Could you check a few things on this drawing? It's one solid part, dimensions in mm from its lowest x, y, z. Round coordinates to 2 decimals unless told otherwise and drop trailing zeros. Write each loop counter-clockwise with the first axis right and the second up, starting at its lowest first coordinate (ties: lowest second). Pieces come first, ordered by that corner, then holes. Notation, with made-up numbers: (66, -23.5) -> (123, -23.5) arc R8 ccw to (123, -13.5) -> close; hole circle Ø4 at (-20, 49). An arc over 180 degrees is marked (long way). Answer as CSV lines item,"result".
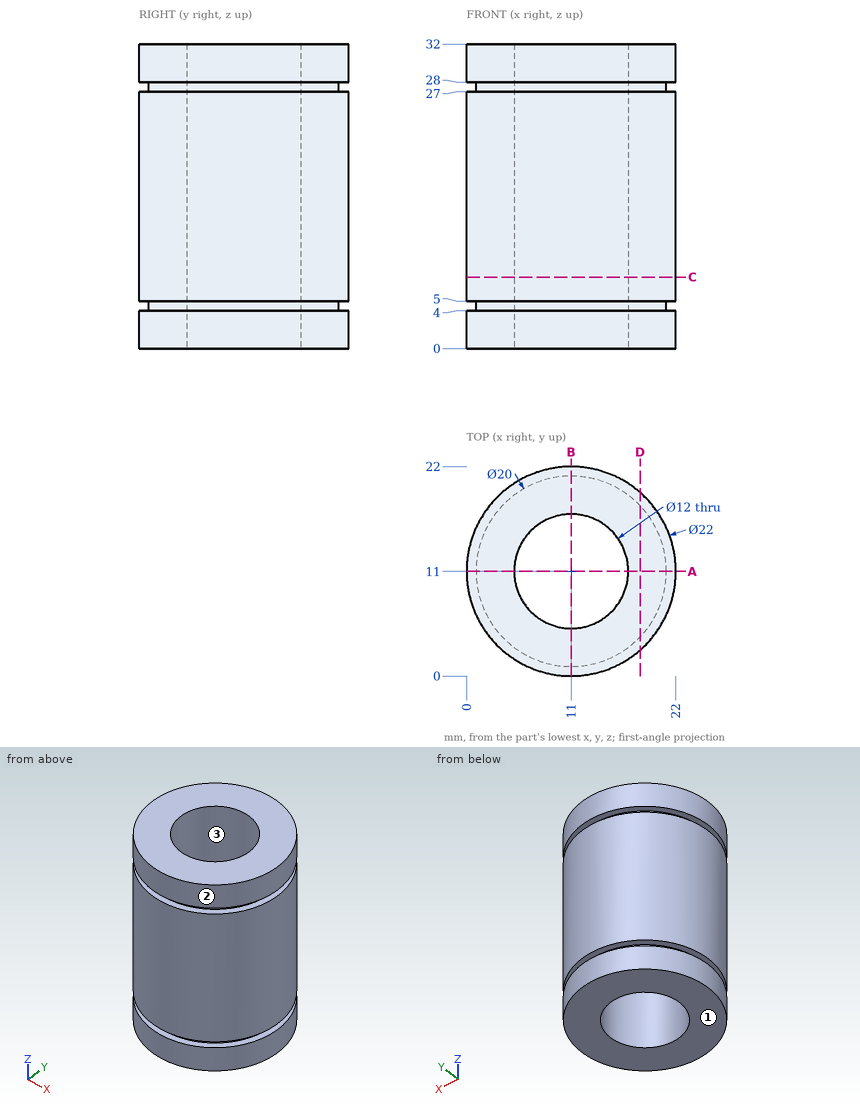
1. For pin 1 Ø12 at (y, z) = (3.5, 9) entering from -X; pin 2 Ø4 at (y, z) = (7, 10.5) entering from +X; pin 3 Ø6.5 at (x, y) = (10, 12) entering from -Z; pin 4 Ø1.5 at (x, z) = (3.5, 25) entering from +Y, each with a flat end and sliding along its axis, tell me the tip position at first contact or that it passes through.
Numbers:
pin 1,"stops at x = 0.1"
pin 2,"stops at x = 21.82"
pin 3,"passes through"
pin 4,"stops at y = 19.69"
2. If I drill on line 1 (Y direction, x = 11, z = 18.5); line 2 (Y direction, x = 15.75, z = 8); line 3 (X direction, y = 6.5, z = 19.5), over which ranges is the centre line in solid material (lowest first)?
Numbers:
line 1,"y = 0 to 5, 17 to 22"
line 2,"y = 1.08 to 7.33, 14.67 to 20.92"
line 3,"x = 0.96 to 7.03, 14.97 to 21.04"
3. If we mould it in two halves opening along X, with no side actions, what happens to the marked faces 1, 2 and 3? For each: released by +X, released by -X, zero draft, split by the parting line, or undercut.
Numbers:
face 1,"zero draft"
face 2,"split by the parting line"
face 3,"undercut"
4. Suppose I cut it at D-D on x = 18.25. Please give me the cut outline in (y, z), and give its area (3 significant figures).
Numbers:
outline,"(2.73, 0) -> (19.27, 0) -> (19.27, 4) -> (17.89, 4) -> (17.89, 5) -> (19.27, 5) -> (19.27, 27) -> (17.89, 27) -> (17.89, 28) -> (19.27, 28) -> (19.27, 32) -> (2.73, 32) -> (2.73, 28) -> (4.11, 28) -> (4.11, 27) -> (2.73, 27) -> (2.73, 5) -> (4.11, 5) -> (4.11, 4) -> (2.73, 4) -> close"
area,"524 mm^2"
5. Suppose I cut it at A-A on y = 11. Please give me the cut outline in (x, z), and give its area (3 significant figures).
Numbers:
outline,"(0, 0) -> (5, 0) -> (5, 32) -> (0, 32) -> (0, 28) -> (1, 28) -> (1, 27) -> (0, 27) -> (0, 5) -> (1, 5) -> (1, 4) -> (0, 4) -> close; (17, 0) -> (22, 0) -> (22, 4) -> (21, 4) -> (21, 5) -> (22, 5) -> (22, 27) -> (21, 27) -> (21, 28) -> (22, 28) -> (22, 32) -> (17, 32) -> close"
area,"316 mm^2"
6. Suppose I cut it at C-C on z = 7.5. Please give me the cut outline in (x, y), and give its area (3 significant figures).
Numbers:
outline,"circle Ø22 at (11, 11); hole circle Ø12 at (11, 11)"
area,"267 mm^2"
